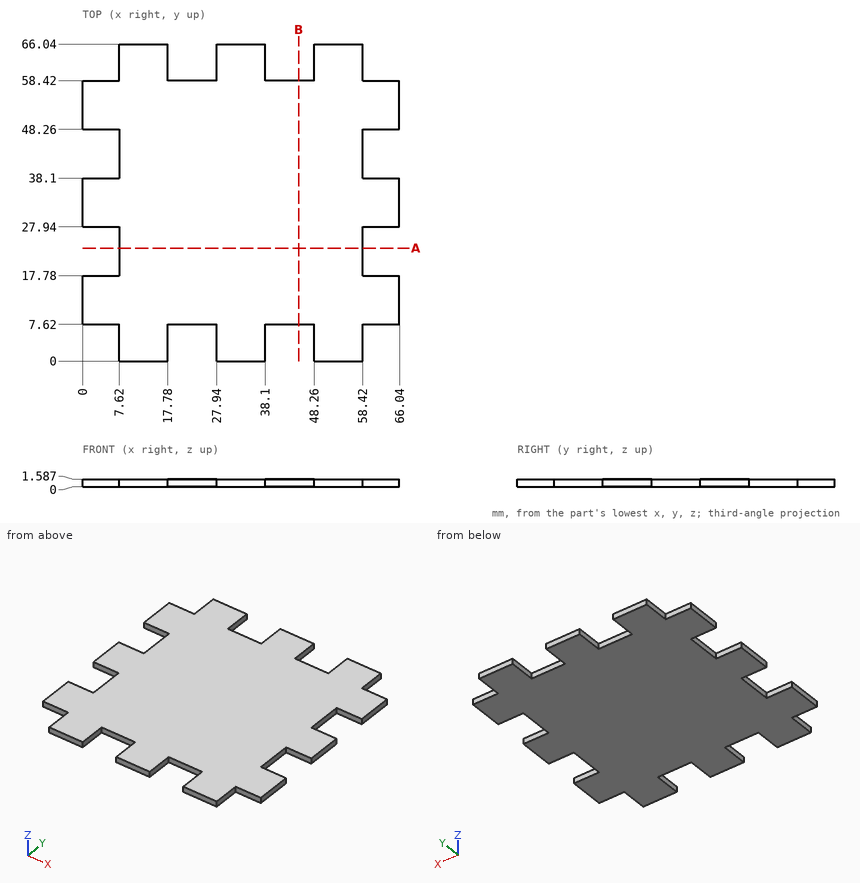
Answer from the drawing. Dimensions are ordinates in mm from the lowest x, y and z of the part. Round coordinates to 2 decimals unless told otherwise and drop trailing zeros. Write each loop counter-clockwise with the first axis right and the second up, starting at its lowest first coordinate (ties: lowest second). Pieces come first, ordered by that corner, then holes.
1. Given pin 1 Ø0.5 at (y, z) = (45.5, 1) entering from -X; pin 2 Ø0.5 at (x, z) = (4.5, 1) entering from +Y; pin 3 Ø0.5 at (y, z) = (62, 0.5) entering from +X, each flat-ended and moving along its own axis, determine where each tip first touches the part or whether it passes through.
2. Straight lines are drawn through the part: L1, parallel to Y at x = 63.5, z = 1.1; L2, parallel to Y at x = 44, z = 1. For each, find the intervals that lie inside material, in ascending order.
3. The part is cut by section A-A, the plane y = 23.5. Determine the outline of the cut face in (x, z).
Values:
1. pin 1: stops at x = 7.62
1. pin 2: stops at y = 58.42
1. pin 3: stops at x = 58.42
2. L1: y = 7.62 to 17.78, 27.94 to 38.1, 48.26 to 58.42
2. L2: y = 7.62 to 58.42
3. outline: (7.62, 0) - (58.42, 0) - (58.42, 1.59) - (7.62, 1.59) - close
